Work out the finished part from the listing and answer in its coordinate system (mm). A direction names the side the tool comes from. Round coordinates to 2 decimals unless told otherwise and drop trailing zeros. Write each loop counter-clockwise with the first axis right and the second up, starting at its lowest first coordinate (ties: lowest second). Pieces come first, ordered by that corner, then holes. Notation, with made-up numbers: M -4.75,-20 L 1.25,-20 A20 cw 1.25,-5 Z; hole C 87,-15 d8. An arc over 180 degrees is marked long. One line per item, written item: value. Start each with the question number.
Q1. The mould has two halves that part along X. Classify faces 1 (the flat face through (-6.15, 2, 0)), 2 (the flat face through (4, 3, -5)), 3 (the flat face through (0, 3, 2.5)), 4 (the flat face through (6.15, 2, 0)): released by +X, released by -X, zero draft, split by the parting line, or undercut.
Q2. Find section C-C (y = 3.2). Write down the section's boundary in (x, z), and give its area (4 significant figures).
Q3. Find section A-A (z = 11.5). Write down the section's boundary in (x, y), and give its area (3 significant figures).
Q4. A tool of negligible diameter and unlimited length cuts with its end or side. For faces 5 (the flat face through (3, 5, 0)), 6 (the flat face through (1.5, 3, -1)), from which of +Z, -Z, +X, -X, +Y, -Y can it reach the whole face along a straight path? Write none if from no direction.
Q5. Given pin 1 Ø1 at (x, z) = (1.5, 9) entering from +Y; pin 2 Ø6 at (x, z) = (5, 11) entering from -Y, each flat-ended and moving along its own axis, determine where each tip first touches the part or whether it passes through.
Q6. Find section D-D (x = 5). Write down the section's boundary in (y, z).
Q7. Consider probe 1 along X at (y, z) = (4.25, 0); probe 2 along X at (y, z) = (3.9, 6.75); probe 3 along Z at (x, y) = (-2.75, 4.6). Determine where each line is inside the solid, lowest interval first.
Q8. Find section B-B (z = -0.5). Write down the section's boundary in (x, y), and give its area (3 significant figures).
from build123d import *

# Parameters (mm, degrees)
SKETCH1_W           = 12.3
SKETCH1_H           = 10
BOSS_EXTRUDE1_DEPTH = 5
SKETCH2_W           = 1.5
SKETCH2_H           = 7.5
CUT_EXTRUDE1_DEPTH  = 5
LPATTERN1_COUNT     = 2
LPATTERN1_PITCH     = 1.5
FILLET4_R           = 0.5
SKETCH3_W           = 0.3
SKETCH3_H           = 0.3
BOSS_EXTRUDE2_DEPTH = 9
SKETCH4_W           = 0.3
SKETCH4_H           = 0.3
BOSS_EXTRUDE3_DEPTH = 7
SKETCH5_W           = 0.3
SKETCH5_H           = 0.3
BOSS_EXTRUDE4_DEPTH = 7
SKETCH6_W           = 0.3
SKETCH6_H           = 0.3
BOSS_EXTRUDE5_DEPTH = 7
SKETCH7_W           = 0.3
SKETCH7_H           = 0.3
BOSS_EXTRUDE6_DEPTH = 7


with BuildPart() as part:
    # Sketch1 → Boss-Extrude1 (new body)
    with BuildSketch(Plane(origin=(0, 0, 0), x_dir=(1, 0, 0), z_dir=(0, 1, 0))):
        Rectangle(SKETCH1_W, SKETCH1_H)
    extrude(amount=BOSS_EXTRUDE1_DEPTH)

    # Sketch2 → Cut-Extrude1 (cut)
    with BuildSketch(Plane(origin=(0, 5, 0), x_dir=(1, 0, 0), z_dir=(0, 1, 0))):
        with Locations((-0.75, 1.25)):
            Rectangle(SKETCH2_W, SKETCH2_H)
    cut_extrude1 = extrude(amount=-CUT_EXTRUDE1_DEPTH, mode=Mode.SUBTRACT)

    # LPattern1: Cut-Extrude1 ×2
    with Locations(*[(i * LPATTERN1_PITCH, 0, 0) for i in range(1, LPATTERN1_COUNT)]):
        add(cut_extrude1, mode=Mode.SUBTRACT)

    # Fillet4
    fillet4_edges = [part.edges().sort_by_distance(p)[0] for p in [
        (-3.825, 0, -5),
        (3.825, 0, -5),
    ]]
    fillet(fillet4_edges, radius=FILLET4_R)

    # Sketch3 → Boss-Extrude2 (add)
    with BuildSketch(Plane.XY.offset(5)):
        with Locations((-4.549701493, 3.935074627)):
            Rectangle(SKETCH3_W, SKETCH3_H)
    extrude(amount=BOSS_EXTRUDE2_DEPTH)

    # Sketch4 → Boss-Extrude3 (add)
    with BuildSketch(Plane.XY.offset(5)):
        with Locations((-4.549701493, 1.340298507)):
            Rectangle(SKETCH4_W, SKETCH4_H)
    extrude(amount=BOSS_EXTRUDE3_DEPTH)

    # Sketch5 → Boss-Extrude4 (add)
    with BuildSketch(Plane.XY.offset(5)):
        with Locations((4.149040482, 3.801410011)):
            Rectangle(SKETCH5_W, SKETCH5_H)
    extrude(amount=BOSS_EXTRUDE4_DEPTH)

    # Sketch6 → Boss-Extrude5 (add)
    with BuildSketch(Plane.XY.offset(5)):
        with Locations((4.149040482, 1.222139303)):
            Rectangle(SKETCH6_W, SKETCH6_H)
    extrude(amount=BOSS_EXTRUDE5_DEPTH)

    # Sketch7 → Boss-Extrude6 (add)
    with BuildSketch(Plane.XY.offset(5)):
        with Locations((3.303641109, 2.378478397)):
            Rectangle(SKETCH7_W, SKETCH7_H)
    extrude(amount=BOSS_EXTRUDE6_DEPTH)


solid = part.part
The answers:
1. face 1: released by -X
1. face 2: zero draft
1. face 3: undercut
1. face 4: released by +X
2. outline: M -6.15,-5 L -1.5,-5 L -1.5,2.5 L 1.5,2.5 L 1.5,-5 L 6.15,-5 L 6.15,5 L -6.15,5 Z
2. area: 100.5 mm2
3. outline: M -4.7,1.19 L -4.4,1.19 L -4.4,1.49 L -4.7,1.49 Z; M -4.7,3.79 L -4.4,3.79 L -4.4,4.09 L -4.7,4.09 Z; M 3.15,2.23 L 3.45,2.23 L 3.45,2.53 L 3.15,2.53 Z; M 4,1.07 L 4.3,1.07 L 4.3,1.37 L 4,1.37 Z; M 4,3.65 L 4.3,3.65 L 4.3,3.95 L 4,3.95 Z
3. area: 0.450 mm2
4. face 5: +Z, -Z, +X, -X, +Y
4. face 6: -Z, +Y, -Y
5. pin 1: through
5. pin 2: y = 1.07
6. outline: M 0,-4.5 A0.5 ccw 0.5,-5 L 5,-5 L 5,5 L 0,5 Z
7. probe 1: -6.15 to -1.5, 1.5 to 6.15
7. probe 2: -4.7 to -4.4, 4 to 4.3
7. probe 3: -5 to 5
8. outline: M -6.15,0 L -1.5,0 L -1.5,5 L -6.15,5 Z; M 1.5,0 L 6.15,0 L 6.15,5 L 1.5,5 Z
8. area: 46.5 mm2
